Model file for the job. Use its own axes, mm. Face numbers are marked on the shaded views. A direction names the side the tool comes from. Give positions to 0.01 mm unless a question says otherwise; leave off trailing zeros. Loops run counter-clockwise (first coordinate to the right, second up) from the corner with the lowest first, then second, coordinate; pieces in that order, holes last. Notation, with made-up numbers: M 28.25,63 L 80.25,63 A34 cw 80.25,100 Z; hole C -39,71 d3. An arc over 180 degrees is marked long. Answer in a Markdown table with one row per item.
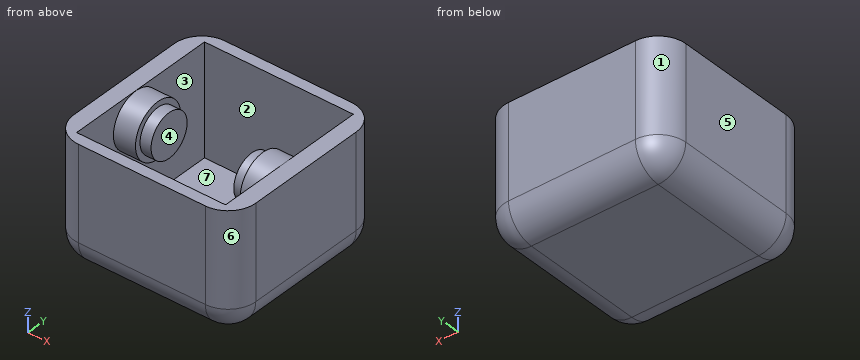
```python
from build123d import *

# Parameters (mm, degrees)
F0_W     = 3
F0_H     = 14
F0_H_2   = 2
F0_W_2   = 27
F0_H_3   = 5
F1_DEPTH = 22
F0_W_3   = 7
F0_H_4   = 10.0040441751
F2_DEPTH = 2
F3_R     = 3.95
F4_DEPTH = 9
F5_R     = 5
F3_R_2   = 4.95
F6_DEPTH = 7


with BuildPart() as f1:
    # F0 (on Top) → F1 (new body)
    with BuildSketch(Plane.XY):
        Polygon((3, 32), (0, 32), (0, 21), (3, 21), (3, 30), align=None)
        Polygon((33, 32), (3, 32), (3, 30), (30, 30), (33, 30), align=None)
        with Locations((31.5, 23)):
            Rectangle(F0_W, F0_H)
        with Locations((31.5, 9)):
            Rectangle(F0_W, F0_H)
        with Locations((31.5, 1)):
            Rectangle(F0_W, F0_H_2)
        with Locations((16.5, 1)):
            Rectangle(F0_W_2, F0_H_2)
        Polygon((3, 11), (0, 11), (0, 0), (3, 0), (3, 2), align=None)
        with Locations((1.5, 13.5)):
            Rectangle(F0_W, F0_H_3)
        with Locations((1.5, 18.5)):
            Rectangle(F0_W, F0_H_3)
    extrude(amount=F1_DEPTH)

    # F0 (on Top) → F2 (join)
    with BuildSketch(Plane.XY):
        Polygon((30, 30), (3, 30), (3, 21), (3, 16), (6.5, 16), (6.5, 26.0040441751), (13.5, 26.0040441751), (13.5, 16), (16.5, 16), (19.5, 16), (19.5, 26.0040441751), (26.5, 26.0040441751), (26.5, 16), (30, 16), align=None)
        Polygon((6.5, 16), (3, 16), (3, 11), (3, 2), (30, 2), (30, 16), (26.5, 16), (26.5, 5.9959558249), (19.5, 5.9959558249), (19.5, 16), (16.5, 16), (13.5, 16), (13.5, 5.9959558249), (6.5, 5.9959558249), align=None)
        with Locations((10, 10.9979779124)):
            Rectangle(F0_W_3, F0_H_4)
        with Locations((10, 21.0020220876)):
            Rectangle(F0_W_3, F0_H_4)
        with Locations((23, 21.0020220876)):
            Rectangle(F0_W_3, F0_H_4)
        with Locations((23, 10.9979779124)):
            Rectangle(F0_W_3, F0_H_4)
    extrude(amount=F2_DEPTH)

    # F3 (on Right) → F4 (join)
    with BuildSketch(Plane.YZ):
        with Locations((15, 17)):
            Circle(F3_R)
    extrude(amount=F4_DEPTH)

    # F5
    f5_edges = [f1.edges().sort_by_distance(p)[0] for p in [
        (16.5, 32, 0),
        (0, 16, 0),
        (16.5, 0, 0),
        (33, 16, 0),
        (33, 32, 11),
        (0, 32, 11),
        (0, 0, 11),
        (33, 0, 11),
    ]]
    fillet(f5_edges, radius=F5_R)

    # F3 (on Right) → F6 (join)
    with BuildSketch(Plane.YZ):
        with Locations((15, 17)):
            Circle(F3_R_2)
        with Locations((15, 17)):
            Circle(F3_R, mode=Mode.SUBTRACT)
    extrude(amount=F6_DEPTH)

    # F8: F1 across plane


with BuildPart() as f1_1:
    add(f1.part)
    add(f1.part.mirror(Plane.YZ.offset(16.5)))


solid = f1_1.part
```
Q1. Saw through at A-A (x = 25). Give the cut face in (y, z).
Reported:
| item | result |
|---|---|
| outline | M 0,5 A5 ccw 5,0 L 27,0 A5 ccw 32,5 L 32,22 L 30,22 L 30,2 L 2,2 L 2,22 L 0,22 Z; C 15,17 d7.9 |
Q2. Saw through at C-C (x = 15). Give the cut face in (y, z).
Reported:
| item | result |
|---|---|
| outline | M 0,5 A5 ccw 5,0 L 27,0 A5 ccw 32,5 L 32,22 L 30,22 L 30,2 L 2,2 L 2,22 L 0,22 Z |
Q3. Mould opens along X. For the marked faces 4, 5, 6 and 7 say: released by +X, released by -X, zero draft, split by the parting line, or undercut.
Reported:
| item | result |
|---|---|
| face 4 | undercut |
| face 5 | released by -X |
| face 6 | released by +X |
| face 7 | undercut |
Q4. Probe probe 1 along X at (y, z) = (24.5, 10.25); probe 2 along Y at (x, z) = (10.5, 8.5); probe 3 along X at (y, z) = (14, 12.5). List the from-to ranges inside material, lowest first.
Reported:
| item | result |
|---|---|
| probe 1 | 0 to 3, 30 to 33 |
| probe 2 | 0 to 2, 30 to 32 |
| probe 3 | 0 to 7, 26 to 33 |
Q5. Saw through at B-B (z = 17). Give the cut face in (x, y), and give its area (3 significant figures).
Reported:
| item | result |
|---|---|
| outline | M 0,5 A5 ccw 5,0 L 28,0 A5 ccw 33,5 L 33,27 A5 ccw 28,32 L 5,32 A5 ccw 0,27 Z; hole M 3,2 L 30,2 L 30,10.05 L 26,10.05 L 26,11.05 L 24,11.05 L 24,18.95 L 26,18.95 L 26,19.95 L 30,19.95 L 30,30 L 3,30 L 3,19.95 L 7,19.95 L 7,18.95 L 9,18.95 L 9,11.05 L 7,11.05 L 7,10.05 L 3,10.05 Z |
| area | 389 mm² |
Q6. Drop a flat-ended pin along its axis: pin 1 (1 mm diameter, centred on x = 21, y = 17.5, fed in from +Z). Give the stop position or say it passes through.
Reported:
| item | result |
|---|---|
| pin 1 | z = 2 |
Q7. Saw through at D-D (y = 24.5). Give the cut face in (x, z).
Reported:
| item | result |
|---|---|
| outline | M 0,5 A5 ccw 5,0 L 28,0 A5 ccw 33,5 L 33,22 L 30,22 L 30,2 L 3,2 L 3,22 L 0,22 Z |
Q8. 3-axis set-ups, long thin cutter, end or side, ignore diameter. For the marked faces 1, 2 and 3: which of +Z, -Z, +X, -X, +Y, -Y reach the whole face in a straight line?
Reported:
| item | result |
|---|---|
| face 1 | +Z, -Z, -X, +Y |
| face 2 | +Z |
| face 3 | none |
